from build123d import *

# Parameters (mm, degrees)
F1_DEPTH = 3.175


with BuildPart() as f1:
    # F0 (on Top) → F1 (new body)
    with BuildSketch(Plane.XY):
        Polygon((-10.4870628137, -6.3373573051), (-5.7407955294, -4.7688256549), (-4.6671820235, -2.8203893327), (-6.8913841292, -2.8648309238), align=None)
        Polygon((-8.1531831795, -9.14692233), (-4.0801120539, -6.2490892989), (-3.6285078717, -4.0707633994), (-5.7407955294, -4.7688256549), align=None)
        Polygon((-4.0801120539, -6.2490892989), (-5.0948574403, -11.1437431653), (-2.056892717, -7.174093935), (-2.267424872, -4.9594322738), align=None)
        Polygon((-0.704871222, -5.4074338266), (-2.056892717, -7.174093935), (-1.583831259, -12.1503935168), (0.1490905642, -7.461648842), align=None)
        Polygon((2.4637240027, -4.8648995948), (2.3418264946, -7.0862035045), (5.5359375832, -10.9313301636), (4.326480864, -6.0811178883), align=None)
        Polygon((3.7882219865, -3.9225703575), (4.326480864, -6.0811178883), (8.512057538, -8.8139355875), (5.9267084221, -4.5356982612), align=None)
        Polygon((4.7761198224, -2.6317035301), (5.9267084221, -4.5356982612), (10.7318438259, -5.9133841552), (7.0003219281, -2.587261939), align=None)
        Polygon((5.3396384525, -1.106998295), (7.0003219281, -2.587261939), (11.998058694, -2.4874025902), (7.4519261103, -0.4089360395), align=None)
        Polygon((5.4287067735, 0.5160685966), (7.4519261103, -0.4089360395), (12.1981933945, 1.1595956107), (7.2413939554, 1.8057256217), align=None)
        Polygon((5.0354106741, 2.0932805287), (7.2413939554, 1.8057256217), (11.314465081, 4.7035586528), (6.3874321692, 3.8599406371), align=None)
        Polygon((4.1946962388, 3.4844952996), (6.3874321692, 3.8599406371), (9.4253968924, 7.8295898674), (4.965919004, 5.5711829878), align=None)
        Polygon((2.9812646346, 4.5660973716), (4.965919004, 5.5711829878), (6.6988408272, 10.2599276626), (3.1031621427, 6.7874012813), align=None)
        Polygon((0.964675707, 7.400529185), (1.5029345845, 5.2419816542), (3.1031621427, 6.7874012813), (3.3770633571, 11.7786258601), align=None)
        Polygon((-0.2447810122, 12.2507414603), (-1.2595263986, 7.3560875939), (-0.1089377989, 5.4520928628), (0.964675707, 7.400529185), align=None)
        Polygon((-3.3718140564, 6.6580253384), (-1.7111305808, 5.1777616944), (-1.2595263986, 7.3560875939), (-3.8448755144, 11.6343249202), align=None)
        Polygon((-7.1033359542, 9.9841475546), (-5.1845012383, 5.3683683133), (-3.1612819015, 4.4433636772), (-3.3718140564, 6.6580253384), align=None)
        Polygon((-9.730633822, 7.446834864), (-6.5365227334, 3.6017082049), (-4.3305394521, 3.3141532979), (-5.1845012383, 5.3683683133), align=None)
        Polygon((-11.4933221725, 4.2478382159), (-7.3077454986, 1.5150205167), (-5.1150095682, 1.8904658542), (-6.5365227334, 3.6017082049), align=None)
        Polygon((-12.2347784104, 0.671402501), (-7.4296430067, -0.706283393), (-5.4449886373, 0.2988022231), (-7.3077454986, 1.5150205167), align=None)
        Polygon((-11.8891208951, -2.9646902726), (-6.8913841292, -2.8648309238), (-5.291156571, -1.3194112967), (-7.4296430067, -0.706283393), align=None)
        Polygon((-6.8913841292, -2.8648309238), (-4.6671820235, -2.8203893327), (-4.0380858348, -1.6786806476), (-5.291156571, -1.3194112967), align=None)
        Polygon((-5.7407955294, -4.7688256549), (-3.6285078717, -4.0707633994), (-3.3638852041, -2.794348271), (-4.6671820235, -2.8203893327), align=None)
        Polygon((-3.6285078717, -4.0707633994), (-4.0801120539, -6.2490892989), (-2.267424872, -4.9594322738), (-2.3907886109, -3.6617257877), align=None)
        Polygon((-2.267424872, -4.9594322738), (-2.056892717, -7.174093935), (-0.704871222, -5.4074338266), (-1.2052599578, -4.2037428989), align=None)
        Polygon((0.0873613318, -4.3722390058), (-0.704871222, -5.4074338266), (0.1490905642, -7.461648842), (0.9203133294, -5.3749611537), align=None)
        Polygon((0.9203133294, -5.3749611537), (0.1490905642, -7.461648842), (2.0679252801, -12.0774280832), (2.3418264946, -7.0862035045), align=None)
        Polygon((1.3722201837, -4.1522424897), (0.9203133294, -5.3749611537), (2.3418264946, -7.0862035045), (2.4637240027, -4.8648995948), align=None)
        Polygon((2.5351512503, -3.5633010067), (2.4637240027, -4.8648995948), (4.326480864, -6.0811178883), (3.7882219865, -3.9225703575), align=None)
        Polygon((3.4728230031, -2.6577445918), (3.7882219865, -3.9225703575), (5.9267084221, -4.5356982612), (4.7761198224, -2.6317035301), align=None)
        Polygon((4.1019191917, -1.5160359067), (4.7761198224, -2.6317035301), (7.0003219281, -2.587261939), (5.3396384525, -1.106998295), align=None)
        Polygon((4.3665418593, -0.2396207783), (5.3396384525, -1.106998295), (7.4519261103, -0.4089360395), (5.4287067735, 0.5160685966), align=None)
        Polygon((4.2431781203, 1.0580857079), (5.4287067735, 0.5160685966), (7.2413939554, 1.8057256217), (5.0354106741, 2.0932805287), align=None)
        Polygon((3.7427893845, 2.2617766355), (5.0354106741, 2.0932805287), (6.3874321692, 3.8599406371), (4.1946962388, 3.4844952996), align=None)
        Polygon((2.9098373869, 3.2644987835), (4.1946962388, 3.4844952996), (4.965919004, 5.5711829878), (2.9812646346, 4.5660973716), align=None)
        Polygon((1.5029345845, 5.2419816542), (1.8183335679, 3.9771558885), (2.9812646346, 4.5660973716), (3.1031621427, 6.7874012813), align=None)
        Polygon((-0.1089377989, 5.4520928628), (0.5652628318, 4.3364252394), (1.5029345845, 5.2419816542), (0.964675707, 7.400529185), align=None)
        Polygon((-1.2595263986, 7.3560875939), (-1.7111305808, 5.1777616944), (-0.7380339876, 4.3103841777), (-0.1089377989, 5.4520928628), align=None)
        Polygon((-3.1612819015, 4.4433636772), (-1.9757532484, 3.9013465659), (-1.7111305808, 5.1777616944), (-3.3718140564, 6.6580253384), align=None)
        Polygon((-5.1845012383, 5.3683683133), (-4.3305394521, 3.3141532979), (-3.0379181626, 3.145657191), (-3.1612819015, 4.4433636772), align=None)
        Polygon((-6.5365227334, 3.6017082049), (-5.1150095682, 1.8904658542), (-3.8301507163, 2.1104623702), (-4.3305394521, 3.3141532979), align=None)
        Polygon((-7.3077454986, 1.5150205167), (-5.4449886373, 0.2988022231), (-4.2820575706, 0.8877437062), (-5.1150095682, 1.8904658542), align=None)
        Polygon((-7.4296430067, -0.706283393), (-5.291156571, -1.3194112967), (-4.3534848183, -0.4138548819), (-5.4449886373, 0.2988022231), align=None)
    extrude(amount=F1_DEPTH)


solid = f1.part
Model file for the job. Use its own axes, mm. A direction names the side the tool comes from. Coordinates: 2 decimals unless noted, no trailing zeros. Write each loop counter-clockwise with the first axis right and the second up, starting at its lowest first coordinate (ties: lowest second). Pieces come first, ordered by that corner, then holes. Notation, with made-up numbers: (40.25, 49.25) -> (82.25, 49.25) arc R16 cw to (82.25, 79.25) -> close; hole circle Ø3 at (63.5, 8.25). An arc over 180 degrees is marked (long way). One line per item, written item: value. Start each with the question number.
1) Flat gauge pins, fed straight in: pin 1 Ø1.5 at (x, z) = (4.5, 0.5) entering from -Y; pin 2 Ø1.5 at (y, z) = (-4, 0.5) entering from -X. Where does each tip first touch, or does it go through?
2) Pull direction X, two halves, no side cores. Call faces 1 (the face through (4.38, 2.18, 1.57)), 2 (the face through (-9.43, 2.9, 1.57)): +X half, -X half, draft (parallel to the pull), parting line (faces both ways), or undercut.
3) Which spindle directions (+Z, -Z, +X, -X, +Y, -Y) get a long thin tool onto all of the face, cutting with end or side? Do faces 3 (the face through (0.37, 9.79, 1.57)), 4 (the face through (-4.69, 1.38, 1.57)), 5 (the face through (3.917, -8.982, 1.565)). Say none if no direction does.
4) Slice it at C-C on x = 9. Write the cut outline in (y, z) (3 decimals), then the cut area to 3 significant figures.
5) Slice it at A-A on x = -8.75. Write the cut outline in (y, z) (1 decimal).
6) Probe probe 1 along Y at (x, z) = (-10, 2.25); probe 2 along X at (y, z) = (-10.5, 0.85); probe 3 along Y at (x, z) = (-6.5, 1.45). List the from-to ranges inside material, lowest first.
7) Slice it at B-B on y = -9.75. Write the cut outline in (x, z) (3 decimals), then the cut area to 3 significant figures.
Answers follow:
1. pin 1: y = -10.59
1. pin 2: x = -8.84
2. face 1: undercut
2. face 2: -X half
3. face 3: +Z, -Z, +Y
3. face 4: +Z, -Z
3. face 5: +Z, -Z, -Y
4. outline: (-5.417, 0) -> (-4.37, 0) -> (-4.37, 3.175) -> (-5.417, 3.175) -> close; (-2.547, 0) -> (-1.117, 0) -> (-1.117, 3.175) -> (-2.547, 3.175) -> close; (0.103, 0) -> (1.576, 0) -> (1.576, 3.175) -> (0.103, 3.175) -> close; (3.057, 0) -> (4.307, 0) -> (4.307, 3.175) -> (3.057, 3.175) -> close; (7.274, 0) -> (7.614, 0) -> (7.614, 3.175) -> (7.274, 3.175) -> close
4. area: 17.6 mm2
5. outline: (-5.8, 0) -> (-4.7, 0) -> (-4.7, 3.2) -> (-5.8, 3.2) -> close; (-2.9, 0) -> (-1.4, 0) -> (-1.4, 3.2) -> (-2.9, 3.2) -> close; (-0.3, 0) -> (1.3, 0) -> (1.3, 3.2) -> (-0.3, 3.2) -> close; (2.5, 0) -> (3.9, 0) -> (3.9, 3.2) -> (2.5, 3.2) -> close; (6.3, 0) -> (7, 0) -> (7, 3.2) -> (6.3, 3.2) -> close
6. probe 1: -6.18 to -5.87, -2.93 to -2.01, 0.03 to 1.05, 3.27 to 4.05
6. probe 2: -4.96 to -4.6, -1.74 to -0.97, 1.41 to 2.15, 5.18 to 5.43
6. probe 3: -7.97 to -6.15, -5.02 to 5.97, 8.53 to 9.45
7. outline: (-4.806, 0) -> (-4.028, 0) -> (-4.028, 3.175) -> (-4.806, 3.175) -> close; (-1.812, 0) -> (-0.697, 0) -> (-0.697, 3.175) -> (-1.812, 3.175) -> close; (1.1, 0) -> (2.196, 0) -> (2.196, 3.175) -> (1.1, 3.175) -> close; (4.555, 0) -> (5.241, 0) -> (5.241, 3.175) -> (4.555, 3.175) -> close
7. area: 11.7 mm2
